Can you work these out from the model? Positions are in its coordinate system, mm. A direction names the side the tool comes from. Give positions to 0.01 mm unless a question says otherwise; leave off trailing zeros. Order: outer loops, then holes, each group sorted by start corner. A loop starts at its lowest first (then second) coordinate and runs counter-clockwise, first axis right, second up. Notation, with made-up numbers: M 14,65.25 L 55,65.25 A33 cw 55,97.25 Z; hole C -4,34 d1. An arc over 180 degrees is marked long. One line per question, with ' | ' between items. Start each with the question number.
1) For faces 1 (the cylindrical face through (13.38, -25.73, 0.69)), 2 (the flat face through (0, 0, -50)), which set-ups out of +Z, -Z, +X, -X, +Y, -Y let a thin tool reach every point of the face, with its end or its side?
2) Please list where these lines run through material, in increasing order: line 1 along Z through (x, y) = (11, 7); line 2 along Y through (x, z) = (0, -8); line 3 along X through (y, z) = (-17, -28). Write a range as [from, to].
3) I'm going to push flat-ended pins straight in: pin 1 Ø6 at (x, z) = (-5.5, -5) entering from +Y; pin 2 Ø8 at (x, z) = (2.5, -22.5) entering from -Y; pin 3 Ø8 at (y, z) = (-4.5, -39) entering from -X. Where does each tip first touch, or does it pass through?
4) If we section it at A-A, the plane y = 0: Please give me the cut outline in (x, z).
5) If we section it at C-C, the plane z = -24.5: Please give me the cut outline in (x, y).
6) Thinking about a two-plate mould opening in Y: for faces 3 (the flat face through (0, 0, 49)), 4 (the cylindrical face through (-29.97, 1.32, 0.7)), 5 (the flat face through (0, 0, 50)), which applies, +Y half, -Y half, draft (parallel to the pull), parting line (faces both ways), or undercut?
```python
from build123d import *

# Parameters (mm, degrees)
F0_R     = 30
F1_DEPTH = 50
F2_R     = 29
F3_DEPTH = 49


with BuildPart() as f1:
    # F0 (on Top) → F1 (new body, symmetric)
    with BuildSketch(Plane.XY):
        Circle(F0_R)
    extrude(amount=F1_DEPTH, both=True)


with BuildPart() as f3:
    # F2 (on Top) → F3 (new body, symmetric)
    with BuildSketch(Plane.XY):
        Circle(F2_R)
    extrude(amount=F3_DEPTH, both=True)


with BuildPart() as f1_1:
    add(f1.part)

    # F4: cut F3
    add(f3.part, mode=Mode.SUBTRACT)


solid = f1_1.part
```
Results found:
1) face 1: none | face 2: -Z, +X, -X, +Y, -Y
2) line 1: z = [-50, -49], [49, 50] | line 2: y = [-30, -29], [29, 30] | line 3: x = [-24.72, -23.49], [23.49, 24.72]
3) pin 1: stops at y = 29.9 | pin 2: stops at y = -30 | pin 3: stops at x = -30
4) outline: M -30,-50 L 30,-50 L 30,50 L -30,50 Z; hole M -29,-49 L 29,-49 L 29,49 L -29,49 Z
5) outline: C 0,0 d60; hole C 0,0 d58
6) face 3: undercut | face 4: parting line | face 5: draft
